```python
from build123d import *

# Parameters (mm, degrees)
BOSS_EXTRUDE1_DEPTH = 3
SKETCH2_W           = 3
SKETCH2_H           = 11.539364706
SKETCH2_H_2         = 9.912138823
SKETCH2_H_3         = 8.2
CUT_EXTRUDE1_DEPTH  = 10
CUT_EXTRUDE2_DEPTH  = 76.2


with BuildPart() as part:
    # Sketch1 → Boss-Extrude1 (new body)
    with BuildSketch(Plane.XY):
        Polygon((0, 0), (0, 20.67), (425, 56.476433126), (425, 39.276433126), align=None)
    extrude(amount=BOSS_EXTRUDE1_DEPTH)

    # Sketch2 → Cut-Extrude1 (cut)
    with BuildSketch(Plane.XY.offset(3)):
        with Locations((17.5, 11.748324541)):
            Rectangle(SKETCH2_W, SKETCH2_H)
        with Locations((216.8, 29.353048358)):
            Rectangle(SKETCH2_W, SKETCH2_H_2)
        with Locations((423.5, 47.876433126)):
            Rectangle(SKETCH2_W, SKETCH2_H_3)
    extrude(amount=-CUT_EXTRUDE1_DEPTH, mode=Mode.SUBTRACT)

    # Sketch4 → Cut-Extrude2 (cut)
    with BuildSketch(Plane.XY.offset(3)):
        with BuildLine():
            Line((28.430075945, 18.586671141), (43.937260326, 19.96620177))
            ThreePointArc((43.937260326, 19.96620177), (50.119919943, 14.793705267), (44.94742344, 8.611045651))
            Line((44.94742344, 8.611045651), (29.440239059, 7.231515022))
            ThreePointArc((29.440239059, 7.231515022), (23.257579443, 12.404011524), (28.430075945, 18.586671141))
        make_face()
        with BuildLine():
            Line((59.790881277, 21.376551653), (78.598406673, 23.049683067))
            ThreePointArc((78.598406673, 23.049683067), (84.78106629, 17.877186565), (79.608569787, 11.694526949))
            Line((79.608569787, 11.694526949), (60.801044391, 10.021395534))
            ThreePointArc((60.801044391, 10.021395534), (54.618384775, 15.193892037), (59.790881277, 21.376551653))
        make_face()
        with BuildLine():
            Line((229.2571326, 36.452395115), (251.2649972, 38.41023108))
            ThreePointArc((251.2649972, 38.41023108), (257.447656816, 33.237734577), (252.275160313, 27.055074961))
            Line((252.275160313, 27.055074961), (230.267295713, 25.097238996))
            ThreePointArc((230.267295713, 25.097238996), (224.084636097, 30.269735499), (229.2571326, 36.452395115))
        make_face()
        with BuildLine():
            Line((93.318457851, 24.359189743), (116.291702582, 26.40290664))
            ThreePointArc((116.291702582, 26.40290664), (122.474362199, 21.230410138), (117.301865696, 15.047750521))
            Line((117.301865696, 15.047750521), (94.328620964, 13.004033624))
            ThreePointArc((94.328620964, 13.004033624), (88.145961348, 18.176530126), (93.318457851, 24.359189743))
        make_face()
        with BuildLine():
            Line((132.414057624, 27.837163307), (155.402232027, 29.88220836))
            ThreePointArc((155.402232027, 29.88220836), (161.584891644, 24.709711857), (156.412395141, 18.527052241))
            Line((156.412395141, 18.527052241), (133.424220738, 16.482007189))
            ThreePointArc((133.424220738, 16.482007189), (127.241561121, 21.654503691), (132.414057624, 27.837163307))
        make_face()
        with BuildLine():
            Line((175.537412929, 31.673448993), (199.853242838, 33.836603264))
            ThreePointArc((199.853242838, 33.836603264), (206.035902455, 28.664106762), (200.863405952, 22.481447145))
            Line((200.863405952, 22.481447145), (176.547576043, 20.318292874))
            ThreePointArc((176.547576043, 20.318292874), (170.364916427, 25.490789377), (175.537412929, 31.673448993))
        make_face()
        with BuildLine():
            Line((276.086850874, 40.618401601), (294.056080345, 42.216957588))
            ThreePointArc((294.056080345, 42.216957588), (300.238739961, 37.044461085), (295.066243459, 30.861801469))
            Line((295.066243459, 30.861801469), (277.097013988, 29.263245482))
            ThreePointArc((277.097013988, 29.263245482), (270.914354371, 34.435741984), (276.086850874, 40.618401601))
        make_face()
        with BuildLine():
            Line((314.592454226, 44.043888646), (335.042833198, 45.863169534))
            ThreePointArc((335.042833198, 45.863169534), (341.225492815, 40.690673031), (336.052996312, 34.508013415))
            Line((336.052996312, 34.508013415), (315.60261734, 32.688732527))
            ThreePointArc((315.60261734, 32.688732527), (309.419957724, 37.86122903), (314.592454226, 44.043888646))
        make_face()
        with BuildLine():
            Line((350.794077228, 47.26441189), (370.423562276, 49.010665445))
            ThreePointArc((370.423562276, 49.010665445), (376.606221893, 43.838168943), (371.43372539, 37.655509326))
            Line((371.43372539, 37.655509326), (351.804240342, 35.909255771))
            ThreePointArc((351.804240342, 35.909255771), (345.621580725, 41.081752274), (350.794077228, 47.26441189))
        make_face()
        with BuildLine():
            Line((385.686896011, 50.36850294), (406.175047046, 52.191144058))
            ThreePointArc((406.175047046, 52.191144058), (412.357706662, 47.018647556), (407.18521016, 40.835987939))
            Line((407.18521016, 40.835987939), (386.697059125, 39.013346821))
            ThreePointArc((386.697059125, 39.013346821), (380.514399509, 44.185843323), (385.686896011, 50.36850294))
        make_face()
    extrude(amount=-CUT_EXTRUDE2_DEPTH, mode=Mode.SUBTRACT)


solid = part.part
```
Source: CAD feature listing. Evaluate the final solid. Frame: model axes, mm. Coordinates: 2 decimals unless noted, no trailing zeros. Loops run counter-clockwise (first coordinate to the right, second up) from the corner with the lowest first, then second, coordinate; pieces in that order, holes last. Notation, with made-up numbers: M 36.25,30 L 83.25,30 A21 cw 83.25,55 Z; hole C 74.25,3 d5. An arc over 180 degrees is marked long. Use a Markdown table: item, result. Add a question column.
Q1. Section query B-B, the plane x = 364.5. Return loops of the section in (y, z), and give its area (3 significant figures).
Q2. Section query A-A, the plane x = 246.5. Return loops of the section in (y, z).
Q3. Material intervals for L1, parallel to Y at x = 101, z = 2.2; L2, parallel to Y at x = 205.5, z = 0.7, sorted ascending.
Q4. Section query C-C, the plane z = 1.1. State how many separate pieces and enclosed holes the cut face has, and give its area (3 significant figures).
Q5. First-contact query: pin 1 (1.5 mm diameter, centred on x = 217.5, z = 1, fed in from +Y); pin 2 (0.9 mm diameter, centred on x = 423.5, z = 1.5, fed in from -Y); pin 3 (1.5 mm diameter, centred on x = 17.5, z = 1.5, fed in from -Y). Flat tips, straight axial feed; report the tip coordinate or a pass-through.
Result:
| question | item | result |
|---|---|---|
| 1 | outline | M 33.69,0 L 37.04,0 L 37.04,3 L 33.69,3 Z; M 48.48,0 L 51.38,0 L 51.38,3 L 48.48,3 Z |
| 1 | area | 18.7 mm2 |
| 2 | outline | M 22.78,0 L 26.54,0 L 26.54,3 L 22.78,3 Z; M 37.99,0 L 41.44,0 L 41.44,3 L 37.99,3 Z |
| 3 | L1 | y = 9.33 to 13.6, 25.04 to 29.18 |
| 3 | L2 | y = 18.99 to 25.7, 30.62 to 37.98 |
| 4 | separate pieces | 1 |
| 4 | enclosed holes | 12 |
| 4 | area | 4,590 mm2 |
| 5 | pin 1 | stops at y = 39.06 |
| 5 | pin 2 | stops at y = 39.1 |
| 5 | pin 3 | stops at y = 1.55 |
